```python
from build123d import *

# Parameters (mm, degrees)
F0_W     = 228.6
F0_H     = 152.4
F1_DEPTH = 76.2
F2_R     = 25.614601
F3_DEPTH = 76.2


with BuildPart() as f1:
    # F0 (on Right) → F1 (new body)
    with BuildSketch(Plane.YZ):
        with Locations((-114.3, 76.2)):
            Rectangle(F0_W, F0_H)
    extrude(amount=F1_DEPTH)

    # F2 (on face) → F3 (cut)
    with BuildSketch(Plane.YZ.offset(76.2)):
        with Locations((-157.394603, 73.01107)):
            Circle(F2_R)
    extrude(amount=-F3_DEPTH, mode=Mode.SUBTRACT)


solid = f1.part
```
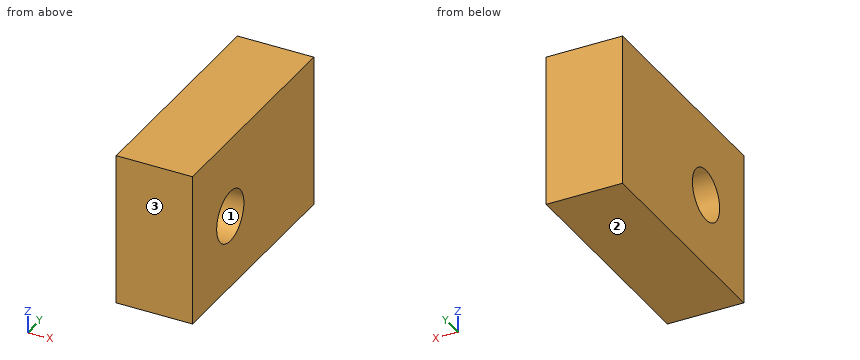
Can you work these out from the model? Positions are in its coordinate system, mm. Face numbers are marked on the shaded views. Give positions to 0.01 mm unless a question says otherwise; leave off trailing zeros. Order: outer loops, then holes, each group sorted by start corner. A loop starts at its lowest first (then second) coordinate and runs counter-clockwise, first axis right, second up. Notation, with made-up numbers: M -13.5,38.25 L 39.5,38.25 A18 cw 39.5,67.25 Z; hole C -12,68.5 d8. An arc over 180 degrees is marked long. Write item = value, one per line. Start each with the question number.
Q1. Suppose I cut it at B-B (x = 63). Write out the boundary of the cut face in (y, z).
Q2. Suppose I cut it at A-A (z = 50). Write out the boundary of the cut face in (x, y).
Q3. We'd pull the mould along Y, two halves only. Please class the marked faces 1, 2 and 3: pulls with the +Y half, pulls with the -Y half, needs draft (parallel to the pull), parting line crosses it, or undercut.
Q4. I need wall thicknesses on probe 1 along Y at (x, z) = (51, 55.5); probe 2 along Z at (x, y) = (25, -134); probe 3 along Y at (x, z) = (12, 78.5). Which ranges of each line are inside material? Lowest first, please. Write a range as [from, to].
Check result:
q1.outline = M -228.6,0 L 0,0 L 0,152.4 L -228.6,152.4 Z; hole C -157.39,73.01 d51.23
q2.outline = M 0,-228.6 L 76.2,-228.6 L 76.2,-168.65 L 0,-168.65 Z; M 0,-146.14 L 76.2,-146.14 L 76.2,0 L 0,0 Z
q3.face_1 = undercut
q3.face_2 = needs draft
q3.face_3 = pulls with the -Y half
q4.probe_1 = [-228.6, -176.09], [-138.7, 0]
q4.probe_2 = [0, 62.58], [83.44, 152.4]
q4.probe_3 = [-228.6, -182.41], [-132.38, 0]
